Design review of the part built by this model. Coordinates are the model's own, in mm. A direction names the side the tool comes from. Coordinates: 2 decimals unless noted, no trailing zeros. Loops run counter-clockwise (first coordinate to the right, second up) from the corner with the lowest first, then second, coordinate; pieces in that order, holes last. Notation, with made-up numbers: (-35, 80.25) -> (-17, 80.25) arc R17 ccw to (-17, 103.25) -> close; hole circle Ø8 at (64, 86.25). An arc over 180 degrees is marked (long way). One line per item, written item: value. Start each with the question number.
1. Draft analysis for pull direction Z (two halves, no side actions). For faces 3 (the flat face through (30.75, 2, 0)), 4 (the cylindrical face through (30.797, 2.486, -22.359)), 5 (the cylindrical face through (-30.797, 2.486, 22.359)), state which applies: pulls with the +Z half, pulls with the -Z half, needs draft (parallel to the pull), parting line crosses it, or undercut.
2. Add section B-B on x = 14.5. Write out the cut boundary in (y, z).
3. Insertion check: pin 1 (5 mm diameter, centred on x = -24, z = 18.5, fed in from +Y). The pin has a flat end and moves straight along its axis. Give the tip position at first contact, or say it passes through.
4. Machinability: for faces 1 (the cylindrical face through (-0.39, 0.54, -23.15)), 2 (the cylindrical face through (-29.609, 1.726, 21.297)), which of the approach directions +Z, -Z, +X, -X, +Y, -Y give a long, thin tool a straight path to every point of the face, cutting with its end or side? Answer none if there is none.
5. For probe 1 along Z at (x, y) = (-17, 3); probe 2 along X at (y, z) = (3.3, -17); probe 3 along Z at (x, y) = (28, 2), list the stretches that pass through material, from the lowest coordinate up.
6. Add section C-C on y = 0.95. Write out the cut boundary in (x, z), plus the area to 3 significant figures.
7. Add section A-A on z = 0.5. Write out the cut boundary in (x, y), plus the area to 3 significant figures.
```python
from build123d import *

# Parameters (mm, degrees)
BOSS_EXTRUDE1_DEPTH = 3.5
FILLET2_R           = 1.5


with BuildPart() as part:
    # Sketch1 → Boss-Extrude1 (new body)
    with BuildSketch(Plane(origin=(0, 0, 0), x_dir=(1, 0, 0), z_dir=(0, 1, 0))):
        with BuildLine():
            Line((-28, 23.5), (28, 23.5))
            ThreePointArc((28, 23.5), (30.828427125, 22.328427125), (32, 19.5))
            Line((32, 19.5), (32, -19.5))
            ThreePointArc((32, -19.5), (30.828427125, -22.328427125), (28, -23.5))
            Line((28, -23.5), (-28, -23.5))
            ThreePointArc((-28, -23.5), (-30.828427125, -22.328427125), (-32, -19.5))
            Line((-32, -19.5), (-32, 19.5))
            ThreePointArc((-32, 19.5), (-30.828427125, 22.328427125), (-28, 23.5))
        make_face()
        with BuildLine():
            Line((-26.75, -22.5), (26.75, -22.5))
            ThreePointArc((26.75, -22.5), (29.578427125, -21.328427125), (30.75, -18.5))
            Line((30.75, -18.5), (30.75, 18.5))
            ThreePointArc((30.75, 18.5), (29.578427125, 21.328427125), (26.75, 22.5))
            Line((26.75, 22.5), (-26.75, 22.5))
            ThreePointArc((-26.75, 22.5), (-29.578427125, 21.328427125), (-30.75, 18.5))
            Line((-30.75, 18.5), (-30.75, -18.5))
            ThreePointArc((-30.75, -18.5), (-29.578427125, -21.328427125), (-26.75, -22.5))
        make_face(mode=Mode.SUBTRACT)
    extrude(amount=BOSS_EXTRUDE1_DEPTH)

    # Fillet2
    # the kernel refuses this fillet: 1.5 mm, written as the material it takes off along each edge
    with BuildSketch(Plane(origin=(-28, 0, -19.5), x_dir=(-1, 0, 0), z_dir=(0, 0, 1))) as fillet2_piece_1:
        with BuildLine():
            CenterArc((4 - FILLET2_R, -FILLET2_R), FILLET2_R, 0, 90)
            Line((4 - FILLET2_R, 0), (4, 0))
            Line((4, 0), (4, -FILLET2_R))
        make_face()
    revolve(axis=Axis((-28, 0, -19.5), (0, -1, 0)), revolution_arc=90, mode=Mode.SUBTRACT)
    with BuildSketch(Plane(origin=(28, 0, -19.5), x_dir=(0, 0, -1), z_dir=(-1, 0, 0))) as fillet2_piece_2:
        with BuildLine():
            CenterArc((4 - FILLET2_R, -FILLET2_R), FILLET2_R, 0, 90)
            Line((4 - FILLET2_R, 0), (4, 0))
            Line((4, 0), (4, -FILLET2_R))
        make_face()
    revolve(axis=Axis((28, 0, -19.5), (0, -1, 0)), revolution_arc=90, mode=Mode.SUBTRACT)
    with BuildSketch(Plane(origin=(28, 0, 19.5), x_dir=(1, 0, 0), z_dir=(0, 0, -1))) as fillet2_piece_3:
        with BuildLine():
            CenterArc((4 - FILLET2_R, -FILLET2_R), FILLET2_R, 0, 90)
            Line((4 - FILLET2_R, 0), (4, 0))
            Line((4, 0), (4, -FILLET2_R))
        make_face()
    revolve(axis=Axis((28, 0, 19.5), (0, -1, 0)), revolution_arc=90, mode=Mode.SUBTRACT)
    with BuildSketch(Plane(origin=(-28, 0, 19.5), x_dir=(0, 0, 1), z_dir=(1, 0, 0))) as fillet2_piece_4:
        with BuildLine():
            CenterArc((4 - FILLET2_R, -FILLET2_R), FILLET2_R, 0, 90)
            Line((4 - FILLET2_R, 0), (4, 0))
            Line((4, 0), (4, -FILLET2_R))
        make_face()
    revolve(axis=Axis((-28, 0, 19.5), (0, -1, 0)), revolution_arc=90, mode=Mode.SUBTRACT)
    with BuildSketch(Plane(origin=(28, 0, 23.5), x_dir=(0, 1, 0), z_dir=(-1, 0, 0)), Plane(origin=(-28, 0, -23.5), x_dir=(0, 1, 0), z_dir=(1, 0, 0))) as fillet2_piece_5:
        with BuildLine():
            CenterArc((FILLET2_R, FILLET2_R), FILLET2_R, 180, 90)
            Line((0, FILLET2_R), (0, 0))
            Line((0, 0), (FILLET2_R, 0))
        make_face()
    extrude(amount=56, mode=Mode.SUBTRACT)
    with BuildSketch(Plane(origin=(-32, 0, 19.5), x_dir=(0, 1, 0), z_dir=(0, 0, -1)), Plane(origin=(32, 0, -19.5), x_dir=(0, 1, 0), z_dir=(0, 0, 1))) as fillet2_piece_6:
        with BuildLine():
            CenterArc((FILLET2_R, FILLET2_R), FILLET2_R, 180, 90)
            Line((0, FILLET2_R), (0, 0))
            Line((0, 0), (FILLET2_R, 0))
        make_face()
    extrude(amount=39, mode=Mode.SUBTRACT)


solid = part.part
```
Worked answers:
1. face 3: undercut
1. face 4: pulls with the -Z half
1. face 5: pulls with the +Z half
2. outline: (0.09, -22.5) arc R1.5 ccw to (1.5, -23.5) -> (3.5, -23.5) -> (3.5, -22.5) -> close; (0.09, 22.5) -> (3.5, 22.5) -> (3.5, 23.5) -> (1.5, 23.5) arc R1.5 ccw to start
3. pin 1: passes through
4. face 1: -Z, +X, -X, -Y
4. face 2: +Y, -Y
5. probe 1: z = -23.5 to -22.5, 22.5 to 23.5
5. probe 2: x = -32 to -30.75, 30.75 to 32
5. probe 3: z = -23.5 to -22.3, 22.3 to 23.5
6. outline: (-31.9, -19.5) arc R3.9 ccw to (-28, -23.4) -> (28, -23.4) arc R3.9 ccw to (31.9, -19.5) -> (31.9, 19.5) arc R3.9 ccw to (28, 23.4) -> (-28, 23.4) arc R3.9 ccw to (-31.9, 19.5) -> close; hole (-30.75, -18.5) arc R4 ccw to (-26.75, -22.5) -> (26.75, -22.5) arc R4 ccw to (30.75, -18.5) -> (30.75, 18.5) arc R4 ccw to (26.75, 22.5) -> (-26.75, 22.5) arc R4 ccw to (-30.75, 18.5) -> close
6. area: 218 mm²
7. outline: (-32, 1.5) arc R1.5 ccw to (-30.75, 0.02) -> (-30.75, 3.5) -> (-32, 3.5) -> close; (30.75, 0.02) arc R1.5 ccw to (32, 1.5) -> (32, 3.5) -> (30.75, 3.5) -> close
7. area: 7.79 mm²
